Geometry: see drawing. Coordinates: mm, zero at the bounding-box minimum. Round coordinates to 2 decimals unless told otherwise and drop trailing zeros. Write each loop counter-clockwise with the first axis right and the second up, starting at its lowest first coordinate (ties: lowest second). Pieces come first, ordered by that corner, then holes. Notation, with made-up numbers: (2, 3) -> (48, 3) arc R30 cw to (48, 40) -> close; hole circle Ø9 at (-28, -10). An arc over 180 degrees is marked (long way). Write item = value, one per line.
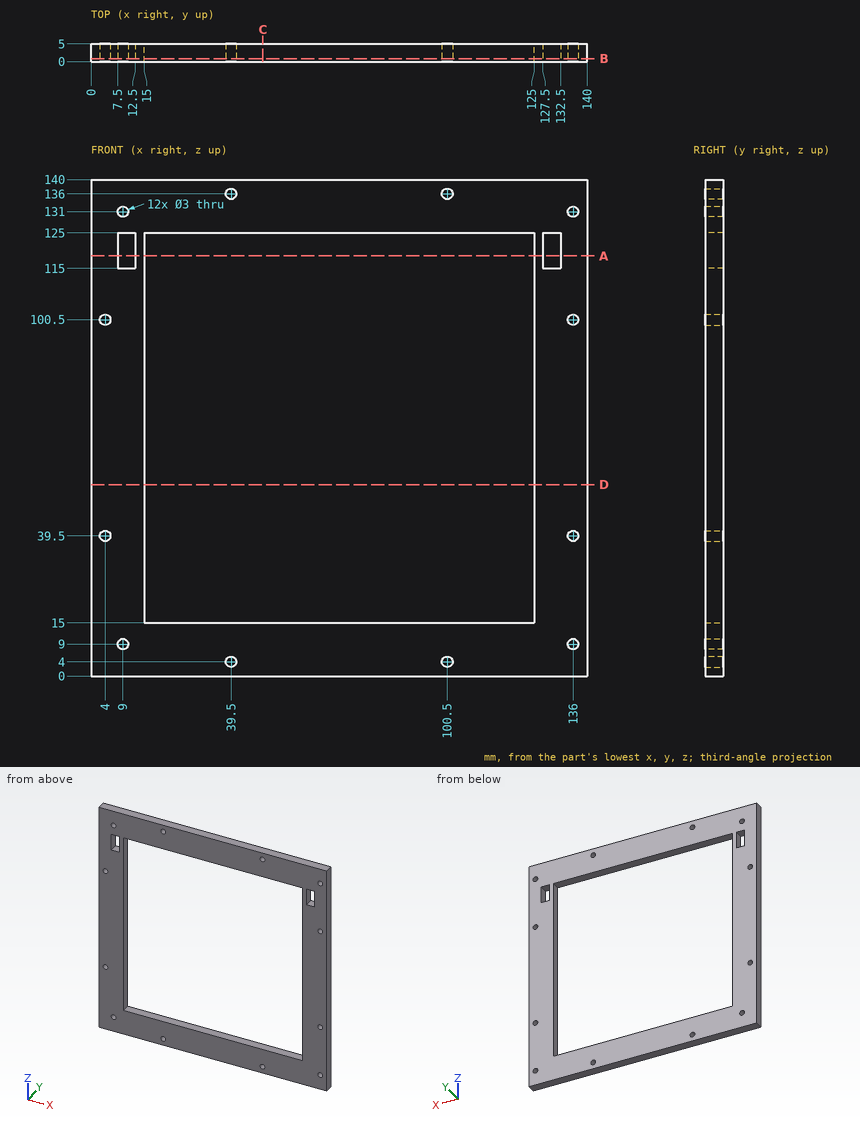
1) First-contact query: P1, Ø2.5, axis at x = 39.5, z = 4, coming from the -Y side. Flat tip, straight axial feed; report the tip coordinate or a pass-through.
Solutions:
P1 = through
2) Cut plane B-B (y = 0.85). Count the separate pieces of the cut face and the enclosed holes in it, and give its area (3 significant figures).
Solutions:
separate_pieces = 1
enclosed_holes = 15
area = 7,320 mm^2
3) Cut plane D-D (z = 54). Return the cut outline in (x, y), and give its area (3 significant figures).
Solutions:
outline = (0, 0) -> (15, 0) -> (15, 5) -> (0, 5) -> close; (125, 0) -> (140, 0) -> (140, 5) -> (125, 5) -> close
area = 150 mm^2
4) Cut plane C-C (x = 48.5). Return the cut outline in (y, z).
Solutions:
outline = (0, 0) -> (5, 0) -> (5, 15) -> (0, 15) -> close; (0, 125) -> (5, 125) -> (5, 140) -> (0, 140) -> close
5) Line query: L1, parallel to Z at x = 100.5, y = 1.95; L2, parallel to X at y = 3, z = 136; L3, parallel to X at y = 4.6, z = 116.5. Output: solid intervals per line, ascending. Write a range as from..to.
Solutions:
L1 = 0..2.5, 5.5..15, 125..134.5, 137.5..140
L2 = 0..38, 41..99, 102..140
L3 = 0..7.5, 12.5..15, 125..127.5, 132.5..140
6) Cut plane A-A (z = 118.5). Return the cut outline in (x, y).
Solutions:
outline = (0, 0) -> (7.5, 0) -> (7.5, 5) -> (0, 5) -> close; (12.5, 0) -> (15, 0) -> (15, 5) -> (12.5, 5) -> close; (125, 0) -> (127.5, 0) -> (127.5, 5) -> (125, 5) -> close; (132.5, 0) -> (140, 0) -> (140, 5) -> (132.5, 5) -> close
